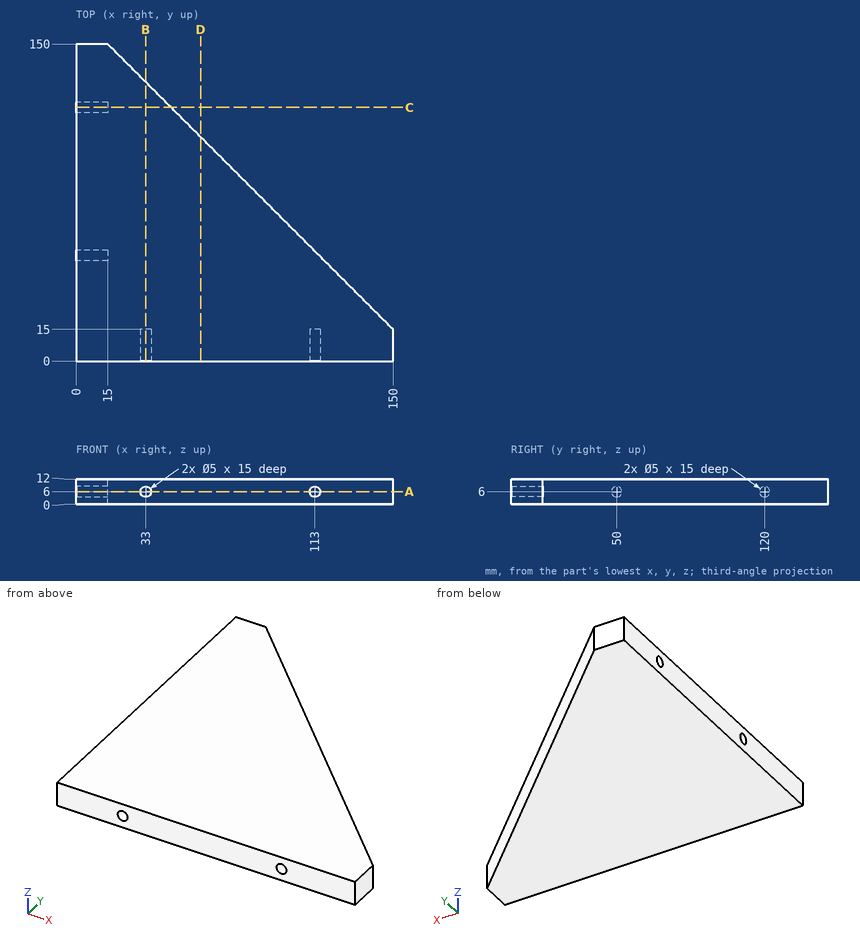
The figure shows three views and two pictorial views of one solid part (mm, origin at its lowest corner). Answer the questions. Give positions to 0.01 mm unless a question says otherwise; leave off trailing zeros. Write each loop counter-clockwise with the first axis right and the second up, starting at its lowest first coordinate (ties: lowest second). Pieces come first, ordered by that corner, then holes. Notation, with made-up numbers: M -32.5,80.25 L 12.5,80.25 A16 ccw 12.5,85.25 Z; hole C 0,-2.75 d4. An arc over 180 degrees is marked long. Write each question's results on one line, items separated by ' | '.
Q1. Section D-D, the plane x = 59 is taken. Write down the section's boundary in (y, z), then the cut area to 3 significant figures.
Output values:
outline: M 0,0 L 106,0 L 106,12 L 0,12 Z | area: 1,270 mm2
Q2. Consider L1, parallel to X at y = 5, z = 6; L2, parallel to Y at x = 11.75, z = 6; L3, parallel to X at y = 8.5, z = 5.25. Determine where each line is inside the solid, lowest interval first. Write a range as from..to.
Output values:
L1: 0..30.5, 35.5..110.5, 115.5..150 | L2: 0..47.5, 52.5..117.5, 122.5..150 | L3: 0..30.62, 35.38..110.62, 115.38..150
Q3. Section A-A, the plane z = 6 is taken. Write down the section's boundary in (x, y), then the cut area to 3 significant figures.
Output values:
outline: M 0,0 L 30.5,0 L 30.5,15 L 35.5,15 L 35.5,0 L 110.5,0 L 110.5,15 L 115.5,15 L 115.5,0 L 150,0 L 150,15 L 15,150 L 0,150 L 0,122.5 L 15,122.5 L 15,117.5 L 0,117.5 L 0,52.5 L 15,52.5 L 15,47.5 L 0,47.5 Z | area: 13,100 mm2
Q4. Flat-ended cylindrical pins translate along their axes: P1, Ø2, axis at x = 68.5, z = 1.5, coming from the +Y side; P2, Ø3, axis at x = 113, z = 6, coming from the -Y side; P3, Ø4.5, axis at x = 33, z = 6, coming from the +Y side. Find the tip coordinate at first contact, or state that the pin passes through.
Output values:
P1: y = 97.5 | P2: y = 15 | P3: y = 134.25
Q5. Section B-B, the plane x = 33 is taken. Write down the section's boundary in (y, z), then the cut area to 3 significant figures.
Output values:
outline: M 0,0 L 132,0 L 132,12 L 0,12 L 0,8.5 L 15,8.5 L 15,3.5 L 0,3.5 Z | area: 1,510 mm2
Q6. Section C-C, the plane y = 120 is taken. Write down the section's boundary in (x, z), then the cut area to 3 significant figures.
Output values:
outline: M 0,0 L 45,0 L 45,12 L 0,12 L 0,8.5 L 15,8.5 L 15,3.5 L 0,3.5 Z | area: 465 mm2
